The model under review builds one solid part; all positions refer to its coordinate system, in mm. Coordinates: 2 decimals unless noted, no trailing zeros. Write each loop counter-clockwise with the first axis right and the second up, starting at its lowest first coordinate (ties: lowest second). Pieces come first, ordered by that corner, then holes. Notation, with made-up numbers: (-5.5, 12) -> (15.5, 12) arc R14 cw to (15.5, 31) -> close; hole circle Ø3 at (67.5, -4.75). An arc over 180 degrees is marked (long way). Put each result on its own line as item: value. Start each with the question number.
from build123d import *

# Parameters (mm, degrees)
SKETCH1_R                  = 43
SKETCH1_R_2                = 36
BOSS_EXTRUDE1_DEPTH        = 0.75
F_3_2_3_2_DIAMETER_HOLE1_D = 3.2


with BuildPart() as part:
    # Sketch1 → Boss-Extrude1 (new body, symmetric)
    with BuildSketch(Plane(origin=(0, 0, 0), x_dir=(1, 0, 0), z_dir=(0, 1, 0))):
        Circle(SKETCH1_R)
        Circle(SKETCH1_R_2, mode=Mode.SUBTRACT)
    extrude(amount=BOSS_EXTRUDE1_DEPTH, both=True)

    # Ø3.2 (3.2) Diameter Hole1 (through all)
    with Locations(Plane(origin=(0, 0.75, 0), x_dir=(1, 0, 0), z_dir=(0, 1, 0))):
        with Locations((-34.208003449, -19.75), (-34.208003449, 19.75), (-19.75, 34.208003449), (19.75, 34.208003449), (34.208003449, 19.75), (34.208003449, -19.75), (19.75, -34.208003449), (-19.75, -34.208003449), (0, 0)):
            Hole(F_3_2_3_2_DIAMETER_HOLE1_D / 2)


solid = part.part
1. Consider section B-B on z = 30.5. State the section outline as (x, y) points, then the cut area to 3 significant figures.
2. Consider section C-C on x = -19.75. State the section outline as (y, z) points.
3. Wall thickness on line 1 (Z direction, x = 0, y = -0.1); line 2 (Z direction, x = -19, y = -0.55); line 3 (Z direction, x = -19.75, y = 0.15): over which ranges is each line inside the solid? List them lowest first. Write a range as from..to.
4. Consider section D-D on y = -0.05. State how many separate pieces and enclosed holes the cut face has, then the cut area to 3 significant figures.
5. Consider section A-A on x = 0. State the section outline as (y, z) points, then the cut area to 3 significant figures.
6. The part is to be moulded in two halves that separate along Z. For faces 1 (the cylindrical face through (-4.686, -0.01, -35.694)), 2 (the cylindrical face through (-5.598, 0.01, -42.634)), 3 (the flat face through (-22.5, 0.75, 28.5)), say which applies: released by +Z, released by -Z, zero draft, split by the parting line, or undercut.
Output values:
1. outline: (-30.31, -0.75) -> (-19.12, -0.75) -> (-19.12, 0.75) -> (-30.31, 0.75) -> close; (19.12, -0.75) -> (30.31, -0.75) -> (30.31, 0.75) -> (19.12, 0.75) -> close
1. area: 33.6 mm^2
2. outline: (-0.75, -38.2) -> (0.75, -38.2) -> (0.75, -35.81) -> (-0.75, -35.81) -> close; (-0.75, -32.61) -> (0.75, -32.61) -> (0.75, -30.1) -> (-0.75, -30.1) -> close; (-0.75, 30.1) -> (0.75, 30.1) -> (0.75, 32.61) -> (-0.75, 32.61) -> close; (-0.75, 35.81) -> (0.75, 35.81) -> (0.75, 38.2) -> (-0.75, 38.2) -> close
3. line 1: z = -43..-36, 36..43
3. line 2: z = -38.57..-35.62, -32.79..-30.58, 30.58..32.79, 35.62..38.57
3. line 3: z = -38.2..-35.81, -32.61..-30.1, 30.1..32.61, 35.81..38.2
4. separate pieces: 1
4. enclosed holes: 9
4. area: 1,670 mm^2
5. outline: (-0.75, -43) -> (0.75, -43) -> (0.75, -36) -> (-0.75, -36) -> close; (-0.75, 36) -> (0.75, 36) -> (0.75, 43) -> (-0.75, 43) -> close
5. area: 21.0 mm^2
6. face 1: undercut
6. face 2: split by the parting line
6. face 3: zero draft
